Could you check a few things on this drawing? It's one solid part, dimensions in mm from its lowest x, y, z. Round coordinates to 2 decimals unless told otherwise and drop trailing zeros. Write each loop counter-clockwise with the first axis right and the second up, starting at its lowest first coordinate (ties: lowest second). Pieces come first, ordered by that corner, then holes. Notation, with made-up numbers: (3.5, 42) - (41.5, 42) arc R11 ccw to (41.5, 60) - close; hole circle Ø3 at (19.25, 39). An arc over 180 degrees is marked (long way). Use one line per item in the form item = value. Start each with the question number.
1. We'd pull the mould along X, two halves only. Please class the marked faces 1, 2 and 3: +X half, -X half, draft (parallel to the pull), parting line (faces both ways), or undercut.
2. I want a section at A-A, the plane z = 142. State how many separate pieces and enclosed holes the cut face has, plus the area to 3 significant figures.
3. I want a section at D-D, the plane x = 88. List the corners of the cut face in (y, z) for me.
4. Will these pins go through, and if not, where does the flat tip stop? pin 1 (10 mm diameter, centred on x = 75.5, z = 23, fed in from +Y); pin 2 (5 mm diameter, centred on x = 170, z = 74.5, fed in from +Y).
5. I want a section at C-C, the plane y = 70.5. List the corners of the cut face in (x, z) for me, plus the area to 3 significant figures.
6. If I drill on line 1 along X through (y, z) = (102, 85); line 2 along Z through (x, y) = (88, 104.15); line 3 along X through (y, z) = (27, 143.5), over which ranges is the centre line in solid material (lowest first)?
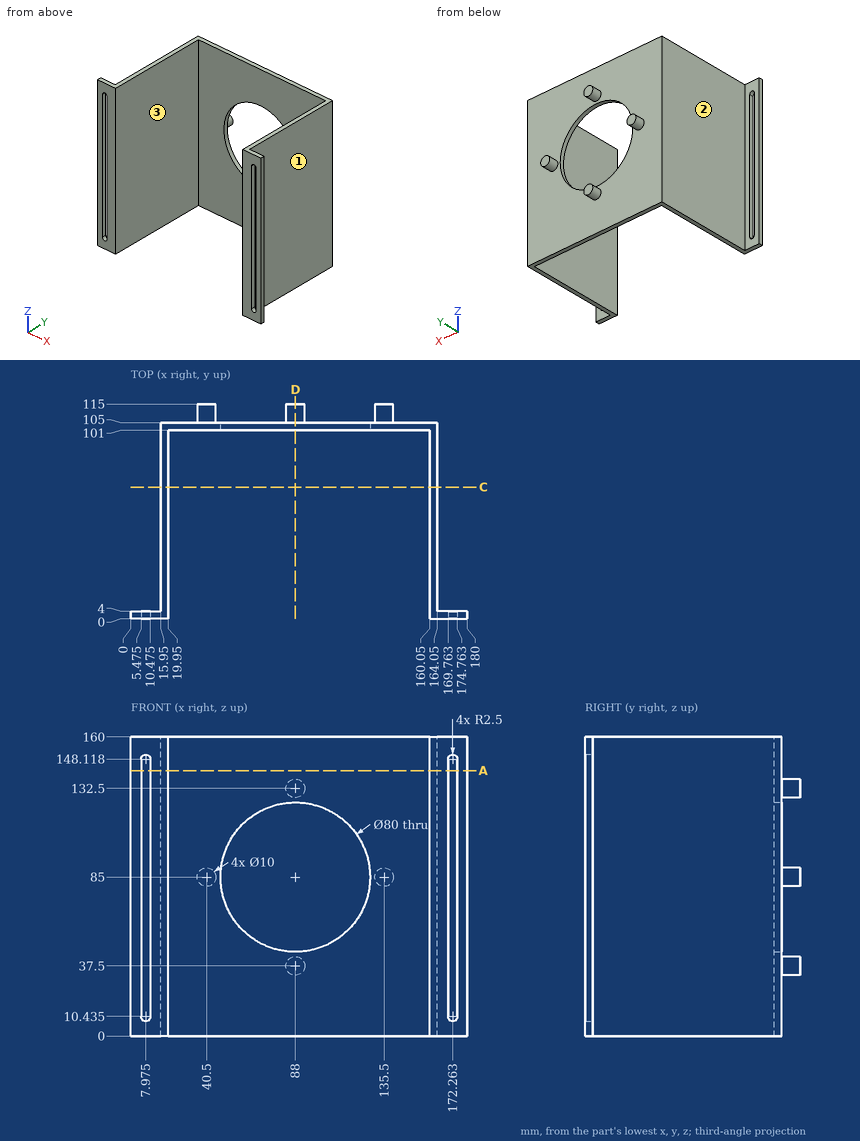
Model answer:
q1.face_1 = +X half
q1.face_2 = -X half
q1.face_3 = undercut
q2.separate_pieces = 3
q2.enclosed_holes = 0
q2.area = 1,490 mm2
q3.outline = (101, 0) - (105, 0) - (105, 32.5) - (115, 32.5) - (115, 42.5) - (105, 42.5) - (105, 45) - (101, 45) - close; (101, 125) - (105, 125) - (105, 127.5) - (115, 127.5) - (115, 137.5) - (105, 137.5) - (105, 160) - (101, 160) - close
q4.pin_1 = 105
q4.pin_2 = 4
q5.outline = (15.95, 0) - (19.95, 0) - (19.95, 160) - (15.95, 160) - close; (160.05, 0) - (164.05, 0) - (164.05, 160) - (160.05, 160) - close
q5.area = 1,280 mm2
q6.line_1 = 15.95 to 48, 128 to 164.05
q6.line_2 = 0 to 45, 125 to 160
q6.line_3 = 15.95 to 19.95, 160.05 to 164.05
